```python
from build123d import *

# Parameters (mm, degrees)
SKETCH1_W           = 34
SKETCH1_H           = 22.65
BOSS_EXTRUDE1_DEPTH = 11.45
SKETCH2_W           = 13.83
SKETCH2_H           = 22.65
BOSS_EXTRUDE2_DEPTH = 24.95
SKETCH5_R           = 1.025
BOSS_EXTRUDE3_DEPTH = 9.86


with BuildPart() as part:
    # Sketch1 → Boss-Extrude1 (new body)
    with BuildSketch(Plane(origin=(0, 0, 0), x_dir=(1, 0, 0), z_dir=(0, 1, 0))):
        Rectangle(SKETCH1_W, SKETCH1_H)
    extrude(amount=BOSS_EXTRUDE1_DEPTH)

    # Sketch2 → Boss-Extrude2 (add)
    with BuildSketch(Plane(origin=(0, 11.45, 0), x_dir=(1, 0, 0), z_dir=(0, 1, 0))):
        with Locations((10.085, 0)):
            Rectangle(SKETCH2_W, SKETCH2_H)
    extrude(amount=BOSS_EXTRUDE2_DEPTH)

    # Sketch5 → Boss-Extrude3 (add)
    with BuildSketch(Plane(origin=(17, 0, 0), x_dir=(0, 0, -1), z_dir=(1, 0, 0))):
        with Locations(Location((0, 27.07, 0), (0, 0, 180))):
            Circle(SKETCH5_R)
    extrude(amount=BOSS_EXTRUDE3_DEPTH)


solid = part.part
```
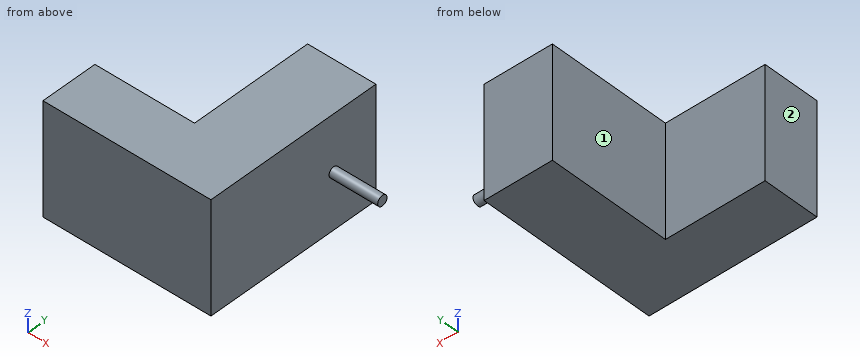
Here's how the part is built. I have some questions about the finished solid (model axes, mm). Face numbers are marked on the shaded views. A direction names the side the tool comes from. Give positions to 0.01 mm unless a question says otherwise; leave off trailing zeros. Write each loop counter-clockwise with the first axis right and the second up, starting at its lowest first coordinate (ties: lowest second). Pieces come first, ordered by that corner, then holes. Notation, with made-up numbers: M 57.5,89 L 101.5,89 A24 ccw 101.5,122 Z; hole C 36.5,52 d11. An arc over 180 degrees is marked long. Put each result on its own line as item: value. Start each with the question number.
Item 1: If we section it at B-B, the plane z = 0: Write out the boundary of the cut face in (x, y) (3 decimals), then the cut area to 3 significant figures.
Item 2: I need wall thicknesses on L1, parallel to Y at x = -8.5, z = 7.25; L2, parallel to X at y = 20, z = 6; L3, parallel to X at y = 7, z = -6. Which ranges of each line are inside material? Lowest first, please. Write a range as from..to.
Item 3: If we section it at A-A, the plane y = 27.07: Write out the boundary of the cut face in (x, z) (3 decimals).
Item 4: If we section it at D-D, the plane z = -9.25: Write out the boundary of the cut face in (x, y).
Item 5: Will these pins go through, and if not, where does the flat tip stop? pin 1 (3 mm diameter, centred on x = -1.5, z = 0, fed in from +Y); pin 2 (8 mm diameter, centred on y = 18.5, z = 7.5, fed in from +X); pin 3 (6 mm diameter, centred on y = 26.5, z = -4.5, fed in from -X).
Item 6: If we section it at C-C, the plane x = 2: Write out the boundary of the cut face in (y, z) (3 decimals), then the cut area to 3 significant figures.
Item 7: On a 3-axis mill with a long thin cutter (end or side, diameter ignored), from which of +Z, -Z, +X, -X, +Y, -Y can I reach the whole of each face in a straight line? I mean the marked faces 1 and 2. Say none if no direction works.
Values:
1. outline: M -17,0 L 17,0 L 17,26.045 L 26.86,26.045 L 26.86,28.095 L 17,28.095 L 17,36.4 L 3.17,36.4 L 3.17,11.45 L -17,11.45 Z
1. area: 755 mm²
2. L1: 0..11.45
2. L2: 3.17..17
2. L3: -17..17
3. outline: M 3.17,-11.325 L 17,-11.325 L 17,-1.025 L 26.86,-1.025 L 26.86,1.025 L 17,1.025 L 17,11.325 L 3.17,11.325 Z
4. outline: M -17,0 L 17,0 L 17,36.4 L 3.17,36.4 L 3.17,11.45 L -17,11.45 Z
5. pin 1: y = 11.45
5. pin 2: x = 17
5. pin 3: x = 3.17
6. outline: M 0,-11.325 L 11.45,-11.325 L 11.45,11.325 L 0,11.325 Z
6. area: 259 mm²
7. face 1: +Z, -Z, -X, +Y
7. face 2: +Z, -Z, -X, +Y, -Y
